```python
from build123d import *

# Parameters (mm, degrees)
SKETCH_1_R      = 2.1
EXTRUDE_1_DEPTH = 100


with BuildPart() as part:
    # 草图1 → 凸台-拉伸1 (new body)
    with BuildSketch(Plane(origin=(0, 0, 0), x_dir=(1, 0, 0), z_dir=(0, 1, 0))):
        with BuildLine():
            Line((8.4, 0), (-8.4, 0))
            ThreePointArc((-8.4, 0), (-9.460660172, 0.439339828), (-9.9, 1.5))
            Line((-9.9, 1.5), (-9.9, 8.4))
            ThreePointArc((-9.9, 8.4), (-9.460660172, 9.460660172), (-8.4, 9.9))
            Line((-8.4, 9.9), (-3.5, 9.9))
            Line((-3.5, 9.9), (-3.5, 9.288498403))
            Line((-3.5, 9.288498403), (-3.2, 9.288498403))
            Line((-3.2, 9.288498403), (-3.2, 8.1))
            Line((-3.2, 8.1), (-6.074788311, 8.1))
            Line((-6.074788311, 8.1), (-6.074788311, 5.792971246))
            Line((-6.074788311, 5.792971246), (-2.616641346, 3.6))
            Line((-2.616641346, 3.6), (2.616641346, 3.6))
            Line((2.616641346, 3.6), (6.074788311, 5.792971246))
            Line((6.074788311, 5.792971246), (6.074788311, 8.1))
            Line((6.074788311, 8.1), (3.2, 8.1))
            Line((3.2, 8.1), (3.2, 9.288498403))
            Line((3.2, 9.288498403), (3.5, 9.288498403))
            Line((3.5, 9.288498403), (3.5, 9.9))
            Line((3.5, 9.9), (8.4, 9.9))
            ThreePointArc((8.4, 9.9), (9.460660172, 9.460660172), (9.9, 8.4))
            Line((9.9, 8.4), (9.9, 1.5))
            ThreePointArc((9.9, 1.5), (9.460660172, 0.439339828), (8.4, 0))
        make_face()
        with Locations(Location((-6.9, 3, 0), (0, 0, 270))):
            Circle(SKETCH_1_R, mode=Mode.SUBTRACT)
        with Locations(Location((6.9, 3, 0), (0, 0, 90))):
            Circle(SKETCH_1_R, mode=Mode.SUBTRACT)
    extrude(amount=EXTRUDE_1_DEPTH)


solid = part.part
```
Work out the finished part from the listing and answer in its coordinate system (mm). A direction names the side the tool comes from. Give positions to 0.01 mm unless a question says otherwise; leave off trailing zeros. Order: outer loops, then holes, each group sorted by start corner. A loop starts at its lowest first (then second) coordinate and runs counter-clockwise, first axis right, second up.
1. The mould has two halves that part along X. Classify faces 4 (the flat face through (4.32, 49.3, -4.68)), 5 (the flat face through (-9.9, 49, -5)), 6 (the flat face through (-6, 49, -9.9)): released by +X, released by -X, zero draft, split by the parting line, or undercut.
Result sheet:
face 4: undercut
face 5: released by -X
face 6: zero draft
2. Each of these flat-tipped pins is pushed along its axis until it touches: P1, Ø1.6, axis at x = 1, y = 50.5, coming from the -Z side; P2, Ø5, axis at x = -6.9, z = -3, coming from the +Y side; P3, Ø1, axis at y = 54.5, z = -9, coming from the +X side; P4, Ø0.7, axis at y = 44.5, z = -9.5, coming from the +X side. Where does it stop, or does it pass through?
Result sheet:
P1: stops at z = -3.6
P2: stops at y = 100
P3: stops at x = 9.9
P4: stops at x = 9.7
3. Section A-A, the plane x = -6.9 is taken. Determine the outline of the cut face in (y, z).
Result sheet:
outline: (0, -9.9) - (100, -9.9) - (100, -5.1) - (0, -5.1) - close; (0, -0.9) - (100, -0.9) - (100, 0) - (0, 0) - close
4. Section B-B, the plane y = 25 is taken. Determine the outline of the cut face in (x, z).
Result sheet:
outline: (-9.9, -8.4) arc R1.5 ccw to (-8.4, -9.9) - (-3.5, -9.9) - (-3.5, -9.29) - (-3.2, -9.29) - (-3.2, -8.1) - (-6.07, -8.1) - (-6.07, -5.79) - (-2.62, -3.6) - (2.62, -3.6) - (6.07, -5.79) - (6.07, -8.1) - (3.2, -8.1) - (3.2, -9.29) - (3.5, -9.29) - (3.5, -9.9) - (8.4, -9.9) arc R1.5 ccw to (9.9, -8.4) - (9.9, -1.5) arc R1.5 ccw to (8.4, 0) - (-8.4, 0) arc R1.5 ccw to (-9.9, -1.5) - close; hole circle Ø4.2 at (-6.9, -3); hole circle Ø4.2 at (6.9, -3)
5. Section C-C, the plane z = -2.5 is taken. Determine the outline of the cut face in (x, y), and give its area (3 significant figures).
Result sheet:
outline: (-9.9, 0) - (-8.94, 0) - (-8.94, 100) - (-9.9, 100) - close; (-4.86, 0) - (4.86, 0) - (4.86, 100) - (-4.86, 100) - close; (8.94, 0) - (9.9, 0) - (9.9, 100) - (8.94, 100) - close
area: 1,160 mm2
6. Straight lines are drawn through the part: L1, parallel to X at y = 56, z = -3; L2, parallel to X at y = 35, z = -4.25; L3, parallel to Z at x = 4.5, y = 19. For each, find the intervals that lie inside material, in ascending order.
Result sheet:
L1: x = -9.9 to -9, -4.8 to 4.8, 9 to 9.9
L2: x = -9.9 to -8.59, -5.21 to -3.64, 3.64 to 5.21, 8.59 to 9.9
L3: z = -9.9 to -8.1, -4.79 to 0
7. For faces 1 (the flat face through (-5, 49, -8.1)), 2 (the flat face through (6, 49, -9.9)), 3 (the flat face through (0, 49, -3.6)), determine the directions among +Z, -Z, +X, -X, +Y, -Y from which every point of the face is accessible in a straight line to the end or side of a thin tool.
Result sheet:
face 1: +Y, -Y
face 2: -Z, +X, -X, +Y, -Y
face 3: -Z, +Y, -Y
8. Section D-D, the plane x = -0.5 is taken. Determine the outline of the cut face in (y, z), and give its area (3 significant figures).
Result sheet:
outline: (0, -3.6) - (100, -3.6) - (100, 0) - (0, 0) - close
area: 360 mm2
